Geometry check sheet. Reference: the model listing, model coordinates, mm. Give positions to 0.01 mm unless a question says otherwise; leave off trailing zeros. Loops run counter-clockwise (first coordinate to the right, second up) from the corner with the lowest first, then second, coordinate; pieces in that order, holes last. Notation, with made-up numbers: (34.5, 44.25) - (57.5, 44.25) arc R11 cw to (57.5, 59.25) - close; hole circle Ø6 at (66, 35.25). An arc over 180 degrees is marked (long way). Write item = value, one per line. Start each with the question number.
from build123d import *

# Parameters (mm, degrees)
EXTRUDE_1_DEPTH     = 10
SKETCH_3_R          = 2
CUT_EXTRUDE_1_DEPTH = 13.328828006
FILLET_2_R          = 0.5


with BuildPart() as part:
    # ｽｹｯﾁ2 → ﾎﾞｽ - 押し出し1 (new body)
    with BuildSketch(Plane.XY):
        Polygon((-6, 4), (6, 4), (2.5, 0), (-2.5, 0), align=None)
    extrude(amount=EXTRUDE_1_DEPTH)

    # ｽｹｯﾁ3 → ｶｯﾄ - 押し出し1 (cut, through all)
    with BuildSketch(Plane(origin=(0, 4, 0), x_dir=(1, 0, 0), z_dir=(0, 1, 0))):
        with Locations(Location((0, -5, 0), (0, 0, 270))):
            Circle(SKETCH_3_R)
    extrude(amount=-CUT_EXTRUDE_1_DEPTH, mode=Mode.SUBTRACT)

    # ﾌｨﾚｯﾄ2
    fillet_2_edges = [part.edges().sort_by_distance(p)[0] for p in [
        (-6, 4, 5),
        (6, 4, 5),
    ]]
    fillet(fillet_2_edges, radius=FILLET_2_R)


solid = part.part
1) Cross-section at B-B on x = 0. Enter the section's corners in (y, z), and give its area (3 significant figures).
2) Gauge pin test, flat end, axial feed: P1, Ø5, axis at x = 0, z = 5, coming from the -Y side. Record the tip position at first contact, or that the pin passes through.
3) Release check for a two-part mould opening along X. For faces 1 (the face through (0, 2, 0)), 2 (the face through (-3.9, 1.6, 4.9)), 3 (the face through (5.35, 3.71, 5.07)), 4 (the face through (0, 2, 3)) record: pulls with the +X half, pulls with the -X half, needs draft (parallel to the pull), parting line crosses it, or undercut.
4) Cross-section at A-A on z = 5. Enter the section's corners in (x, y).
5) Cross-section at C-C on y = 0.4. Enter the section's corners in (x, z).
6) Cross-section at D-D on z = 8. Enter the section's corners in (x, y), and give its area (3 significant figures).
7) Material ranges on line 1 along X through (y, z) = (1.85, 5); line 2 along X through (y, z) = (2, 5); line 3 along Z through (x, y) = (0.5, 2.6), recorded low to high.
Checked values:
q1.outline = (0, 0) - (4, 0) - (4, 3) - (0, 3) - close; (0, 7) - (4, 7) - (4, 10) - (0, 10) - close
q1.area = 24.0 mm²
q2.P1 = 0
q3.face_1 = needs draft
q3.face_2 = pulls with the -X half
q3.face_3 = pulls with the +X half
q3.face_4 = undercut
q4.outline = (-5.27, 3.17) - (-2.5, 0) - (-2, 0) - (-2, 4) - (-4.9, 4) arc R0.5 ccw to start; (2, 0) - (2.5, 0) - (5.27, 3.17) arc R0.5 ccw to (4.9, 4) - (2, 4) - close
q5.outline = (-2.85, 0) - (2.85, 0) - (2.85, 10) - (-2.85, 10) - close; hole circle Ø4 at (0, 5)
q6.outline = (-5.27, 3.17) - (-2.5, 0) - (2.5, 0) - (5.27, 3.17) arc R0.5 ccw to (4.9, 4) - (-4.9, 4) arc R0.5 ccw to start
q6.area = 33.5 mm²
q7.line_1 = -4.12 to -2, 2 to 4.12
q7.line_2 = -4.25 to -2, 2 to 4.25
q7.line_3 = 0 to 3.06, 6.94 to 10
